```python
from build123d import *

# Parameters (mm, degrees)
SKETCH1_R           = 101.6
BOSS_EXTRUDE1_DEPTH = 3.175
SKETCH2_R           = 12.827
CUT_EXTRUDE1_DEPTH  = 3.175
SKETCH3_R           = 63.5
CUT_EXTRUDE2_DEPTH  = 4.175


with BuildPart() as part:
    # Sketch1 → Boss-Extrude1 (new body)
    with BuildSketch(Plane(origin=(0, 0, 0), x_dir=(1, 0, 0), z_dir=(0, 1, 0))):
        Circle(SKETCH1_R)
    extrude(amount=BOSS_EXTRUDE1_DEPTH)

    # Sketch2 → Cut-Extrude1 (cut)
    with BuildSketch(Plane(origin=(0, 3.175, 0), x_dir=(1, 0, 0), z_dir=(0, 1, 0))):
        with Locations((0, 82.55)):
            Circle(SKETCH2_R)
        with Locations((78.50971542, 25.509352886)):
            Circle(SKETCH2_R)
        with Locations((48.521672577, -66.784352886)):
            Circle(SKETCH2_R)
        with Locations((-48.521672577, -66.784352886)):
            Circle(SKETCH2_R)
        with Locations((-78.50971542, 25.509352886)):
            Circle(SKETCH2_R)
    extrude(amount=-CUT_EXTRUDE1_DEPTH, mode=Mode.SUBTRACT)

    # Sketch3 → Cut-Extrude2 (cut, through all)
    with BuildSketch(Plane(origin=(0, 3.175, 0), x_dir=(1, 0, 0), z_dir=(0, 1, 0))):
        Circle(SKETCH3_R)
    extrude(amount=-CUT_EXTRUDE2_DEPTH, mode=Mode.SUBTRACT)


solid = part.part
```
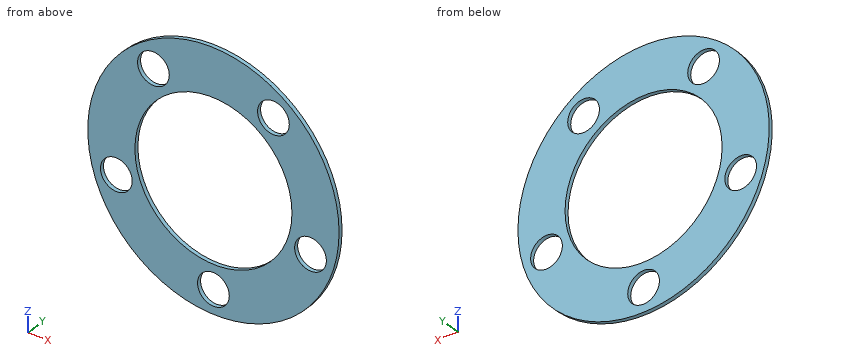
Design review of the part built by this model. Coordinates are the model's own, in mm. Coordinates: 2 decimals unless noted, no trailing zeros. Write each loop counter-clockwise with the first axis right and the second up, starting at its lowest first coordinate (ties: lowest second). Pieces come first, ordered by that corner, then holes.
1) Add section B-B (z = 0). Write out the cut boundary in (x, y) (3 decimals).
2) Add section D-D (x = 85). Write out the cut boundary in (y, z) (3 decimals).
3) Insertion check: pin 1 (1.5 mm diameter, centred on x = 32, y = 0.5, fed in from +Z); pin 2 (20.5 mm diameter, centred on x = 78.51, z = -25.51, fed in from -Y); pin 3 (1 mm diameter, centred on y = 1, z = -30, fed in from +X). Each pin has a flat end and moves straight along its axis. Give the tip position at first contact, or say it passes through.
4) Add section A-A (x = 0). Write out the cut boundary in (y, z) (3 decimals).
5) To check wall thickness, follow L1, parallel to Z at x = 0, y = 0.9; L2, parallel to Z at x = 8, y = 1.95; L3, parallel to X at y = 1.1, z = 0. State the ranges of each line that lie inside material, in increasing order.
6) Add section C-C (y = 2.55). Write out the cut boundary in (x, z), plus the area to 3 significant figures.
Check result:
1. outline: (-101.6, 0) - (-63.5, 0) - (-63.5, 3.175) - (-101.6, 3.175) - close; (63.5, 0) - (101.6, 0) - (101.6, 3.175) - (63.5, 3.175) - close
2. outline: (0, -55.656) - (3.175, -55.656) - (3.175, -36.573) - (0, -36.573) - close; (0, -14.446) - (3.175, -14.446) - (3.175, 55.656) - (0, 55.656) - close
3. pin 1: stops at z = 96.67
3. pin 2: passes through
3. pin 3: stops at x = 97.22
4. outline: (0, -101.6) - (3.175, -101.6) - (3.175, -95.377) - (0, -95.377) - close; (0, -69.723) - (3.175, -69.723) - (3.175, -63.5) - (0, -63.5) - close; (0, 63.5) - (3.175, 63.5) - (3.175, 101.6) - (0, 101.6) - close
5. L1: z = -101.6 to -95.38, -69.72 to -63.5, 63.5 to 101.6
5. L2: z = -101.28 to -92.58, -72.52 to -62.99, 62.99 to 101.28
5. L3: x = -101.6 to -63.5, 63.5 to 101.6
6. outline: circle Ø203.2 at (0, 0); hole circle Ø25.65 at (-78.51, -25.51); hole circle Ø127 at (0, 0); hole circle Ø25.65 at (-48.52, 66.78); hole circle Ø25.65 at (0, -82.55); hole circle Ø25.65 at (48.52, 66.78); hole circle Ø25.65 at (78.51, -25.51)
6. area: 17,200 mm2
